from build123d import *

# Parameters (mm, degrees)
F0_R            = 3.175
F1_DEPTH        = 2
F3_DEPTH        = 2.001
F3_COPIES_COUNT = 4


# Not quite as in the source:
# - a pattern or mirror of a feature is missing from the dataset's text; its kind, count and spacing are read off the source's solid


with BuildPart() as f1:
    # F0 (on Top) → F1 (new body)
    with BuildSketch(Plane.XY):
        with BuildLine():
            Line((-84.6666666667, -23.9473496562), (-16.9333333333, -47.8946993124))
            ThreePointArc((-16.9333333333, -47.8946993124), (50.8, 0), (-16.9333333333, 47.8946993124))
            Line((-16.9333333333, 47.8946993124), (-84.6666666667, 23.9473496562))
            ThreePointArc((-84.6666666667, 23.9473496562), (-101.6, 0), (-84.6666666667, -23.9473496562))
        make_face()
        with Locations((-76.2, 0)):
            Circle(F0_R, mode=Mode.SUBTRACT)
        Circle(F0_R, mode=Mode.SUBTRACT)
    extrude(amount=F1_DEPTH)

    # F2 (on face) → F3 (cut, through all)
    with BuildSketch(Plane.XY.offset(2)):
        with BuildLine():
            ThreePointArc((-28.7020344674, -19.8984633183), (-34.6367957344, -4.4775), (-32.8185304223, 11.945697381))
            ThreePointArc((-32.8185304223, 11.945697381), (-44.5595640794, 7.3696726522), (-45.9028628242, -5.1597895126))
            Line((-45.9028628242, -5.1597895126), (-40.9229625402, -15.7549236864))
            ThreePointArc((-40.9229625402, -15.7549236864), (-35.6939675857, -20.4264925159), (-28.7020344674, -19.8984633183))
        make_face()
        with BuildLine():
            ThreePointArc((-22.8444099031, -1.093728902), (-25.2904359206, 7.3696726522), (-32.8185304223, 11.945697381))
            ThreePointArc((-32.8185304223, 11.945697381), (-34.6367957344, -4.4775), (-28.7020344674, -19.8984633183))
            ThreePointArc((-28.7020344674, -19.8984633183), (-25.386046138, -16.940715135), (-23.9000073953, -12.7531452225))
            Line((-23.9000073953, -12.7531452225), (-22.8444099031, -1.093728902))
        make_face()
    f3 = extrude(amount=-F3_DEPTH, mode=Mode.SUBTRACT)

    # F3_copies: F3 ×4 about axis
    f3_copies_axis = Axis((0, 0, 0), (0, 0, 1))
    for i in range(1, F3_COPIES_COUNT):
        add(f3.rotate(f3_copies_axis, i * 360 / F3_COPIES_COUNT), mode=Mode.SUBTRACT)


solid = f1.part
Design review of the part built by this model. Coordinates are the model's own, in mm. A direction names the side the tool comes from. Coordinates: 2 decimals unless noted, no trailing zeros. Write each loop counter-clockwise with the first axis right and the second up, starting at its lowest first coordinate (ties: lowest second). Pieces come first, ordered by that corner, then holes. Notation, with made-up numbers: (80, 38) -> (117, 38) arc R20 ccw to (117, 67) -> close; hole circle Ø4 at (-9.5, 2). An arc over 180 degrees is marked (long way). Write each question's results on one line, items separated by ' | '. Start each with the question number.
(1) Tool access review of faces 5 (the face through (43.45, 10.38, 1.01)), 6 (the face through (-51.274, -35.753, 0.986)): name each direction out of +Z, -Z, +X, -X, +Y, -Y from which nothing blocks a thin tool from reaching the whole face with its end or side.
(2) For line 1 along X through (y, z) = (2.5, 1.7); line 2 along X through (y, z) = (-6.5, 0.7); line 3 along X through (y, z) = (-7.5, 0.6), list the stretches that pass through material, from the lowest coordinate up. Write a range as from..to.
(3) Take a section at D-D on y = 7.5. Write out the cut boundary in (x, z).
(4) Clearance check with a flat-ended pin moving along its axis: P1, Ø4, axis at x = 0, y = 0, coming from the +Z side. State where the tip first meets the part, or that it passes through.
(5) Take a section at B-B on x = -76.2. Write out the cut boundary in (y, z) (3 decimals).
(6) Take a section at A-A on z = 1.1. Write out the cut boundary in (x, y) (3 decimals), and give its area (3 significant figures).
(7) Take a section at C-C on y = -38.5. Write out the cut boundary in (x, z).
(8) The part is to be moulded in two halves that separate along Y. For faces 1 (the face through (-73.17, 0.95, 0.99)), 2 (the face through (50.78, -1.36, 0.99)), 3 (the face through (-26, 12, 2)), 4 (the face through (-50.326, 36.089, 0.986)), say which applies: pulls with the +Y half, pulls with the -Y half, needs draft (parallel to the pull), parting line crosses it, or undercut.
Results found:
1) face 5: +Z, -Z | face 6: +Z, -Z, -X, -Y
2) line 1: x = -101.48..-78.16, -74.24..-46.79, -23.06..-1.96, 1.96..22.97, 46.79..50.74 | line 2: x = -100.75..-45.27, -23.33..24.68, 45.17..50.38 | line 3: x = -100.47..-44.8, -23.42..25.39, 44.46..50.24
3) outline: (-100.47, 0) -> (-44.46, 0) -> (-44.46, 2) -> (-100.47, 2) -> close; (-25.39, 0) -> (23.42, 0) -> (23.42, 2) -> (-25.39, 2) -> close; (44.8, 0) -> (50.24, 0) -> (50.24, 2) -> (44.8, 2) -> close
4) P1: passes through
5) outline: (-26.941, 0) -> (-3.175, 0) -> (-3.175, 2) -> (-26.941, 2) -> close; (3.175, 0) -> (26.941, 0) -> (26.941, 2) -> (3.175, 2) -> close
6) outline: (-84.667, -23.947) -> (-16.933, -47.895) arc R50.8 ccw (long way) to (-16.933, 47.895) -> (-84.667, 23.947) arc R25.4 ccw to start; hole circle Ø6.35 at (-76.2, 0); hole (-45.903, -5.16) -> (-40.923, -15.755) arc R8.955 ccw to (-23.9, -12.753) -> (-22.844, -1.094) arc R12.13 ccw (long way) to start; hole (-15.755, 40.923) arc R8.955 ccw to (-12.753, 23.9) -> (-1.094, 22.844) arc R12.13 ccw (long way) to (-5.16, 45.903) -> close; hole circle Ø6.35 at (0, 0); hole (1.094, -22.844) arc R12.13 ccw (long way) to (5.16, -45.903) -> (15.755, -40.923) arc R8.955 ccw to (12.753, -23.9) -> close; hole (22.844, 1.094) arc R12.13 ccw (long way) to (45.903, 5.16) -> (40.923, 15.755) arc R8.955 ccw to (23.9, 12.753) -> close | area: 8,650 mm2
7) outline: (-43.51, 0) -> (-11.59, 0) -> (-11.59, 2) -> (-43.51, 2) -> close; (18.87, 0) -> (33.14, 0) -> (33.14, 2) -> (18.87, 2) -> close
8) face 1: undercut | face 2: parting line crosses it | face 3: needs draft | face 4: pulls with the +Y half
